Study the drawing (mm; zero at the part's minimum x, y, z) and answer. Coordinates: 2 decimals unless noted, no trailing zeros. Write each loop counter-clockwise with the first axis right and the second up, starting at its lowest first coordinate (ties: lowest second). Pieces come first, ordered by that corner, then holes. Notation, with made-up numbers: M 26,2.5 L 48,2.5 A35 ccw 48,38.5 Z; hole C -20.75,-5 d4. An arc over 180 degrees is marked long. Answer as a JSON object with one key per item and string values. Group by question number.
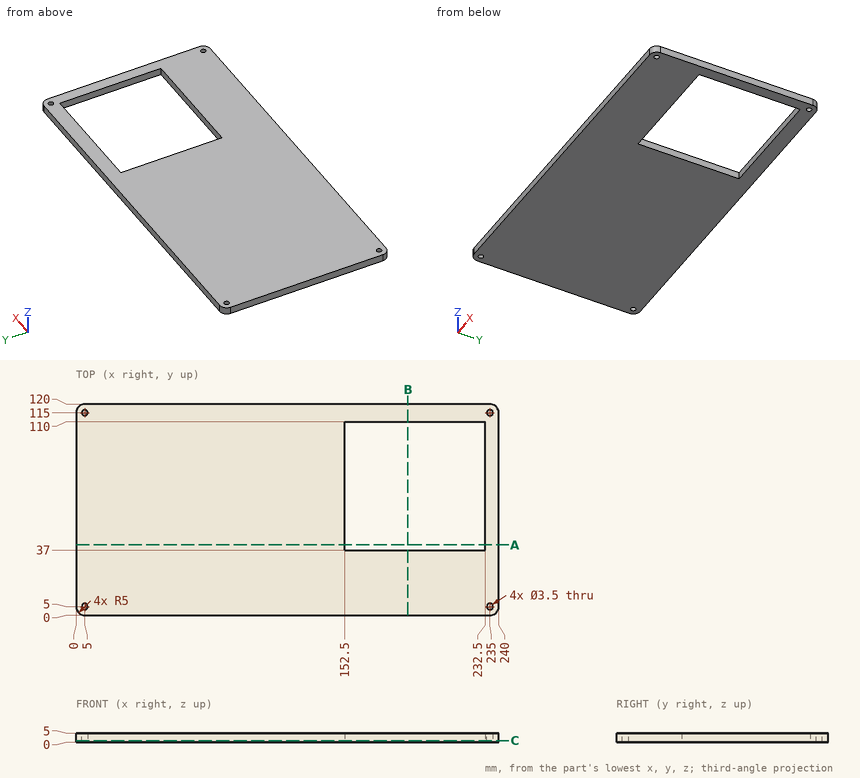
Item 1: A cutting plane is placed at C-C, the plane z = 0.8. Write down the section's boundary in (x, y).
Item 2: Consider L1, parallel to Y at x = 235, z = 2.35; L2, parallel to X at y = 115, z = 3; L3, parallel to Y at x = 177, z = 2.7. Determine where each line is inside the solid, lowest interval first. Write a range as from..to.
Item 3: A cutting plane is placed at A-A, the plane y = 40. Write down the section's boundary in (x, z), and give its area (3 significant figures).
Item 4: A cutting plane is placed at B-B, the plane x = 188.5. Write down the section's boundary in (y, z).
Answer:
{
 "1": {"outline": "M 0,5 A5 ccw 5,0 L 235,0 A5 ccw 240,5 L 240,115 A5 ccw 235,120 L 5,120 A5 ccw 0,115 Z; hole C 5,5 d3.5; hole C 5,115 d3.5; hole M 152.5,37 L 232.5,37 L 232.5,110 L 152.5,110 Z; hole C 235,5 d3.5; hole C 235,115 d3.5"},
 "2": {"L1": "0..3.25, 6.75..113.25, 116.75..120", "L2": "0..3.25, 6.75..233.25, 236.75..240", "L3": "0..37, 110..120"},
 "3": {"outline": "M 0,0 L 152.5,0 L 152.5,5 L 0,5 Z; M 232.5,0 L 240,0 L 240,5 L 232.5,5 Z", "area": "800 mm2"},
 "4": {"outline": "M 0,0 L 37,0 L 37,5 L 0,5 Z; M 110,0 L 120,0 L 120,5 L 110,5 Z"}
}
